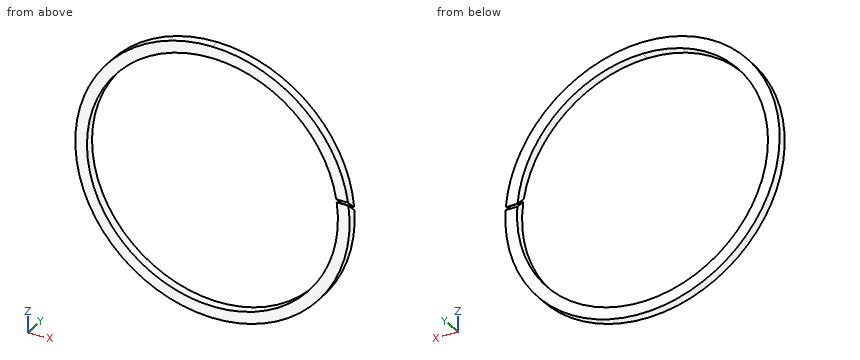
from build123d import *

# Parameters (mm, degrees)
SKETCH1_R           = 47
SKETCH1_R_2         = 43
BOSS_EXTRUDE1_DEPTH = 3
CUT_EXTRUDE1_DEPTH  = 10


with BuildPart() as part:
    # Sketch1 → Boss-Extrude1 (new body)
    with BuildSketch(Plane(origin=(0, 0, 0), x_dir=(1, 0, 0), z_dir=(0, 1, 0))):
        with Locations(Location((0, 0, 0), (0, 0, 270))):
            Circle(SKETCH1_R)
        with Locations(Location((0, 0, 0), (0, 0, 270))):
            Circle(SKETCH1_R_2, mode=Mode.SUBTRACT)
    extrude(amount=BOSS_EXTRUDE1_DEPTH)

    # Sketch3 → Cut-Extrude1 (cut)
    with BuildSketch(Plane(origin=(47, 0, 0), x_dir=(0, 0, -1), z_dir=(1, 0, 0))):
        Polygon((-4, 3), (-7, 0), (-6, 0), (-3, 3), align=None)
    extrude(amount=-CUT_EXTRUDE1_DEPTH, mode=Mode.SUBTRACT)


solid = part.part
Part model, mm, in its own coordinate system. Coordinates: 2 decimals unless noted, no trailing zeros. Order: outer loops, then holes, each group sorted by start corner. A loop starts at its lowest first (then second) coordinate and runs counter-clockwise, first axis right, second up.
(1) Slice it at B-B, the plane x = -37. Write the cut outline in (y, z).
Check sheet entries:
outline: (0, -28.98) - (3, -28.98) - (3, -21.91) - (0, -21.91) - close; (0, 21.91) - (3, 21.91) - (3, 28.98) - (0, 28.98) - close
(2) Slice it at C-C, the plane y = 2.1. Write the cut outline in (x, z), and give its area (3 significant figures).
Check sheet entries:
outline: (42.72, 4.9) - (46.74, 4.9) arc R47 ccw (long way) to (46.84, 3.9) - (42.82, 3.9) arc R43 cw (long way) to start
area: 1,130 mm2
(3) Probe L1, parallel to Z at x = 0, y = 2.4; L2, parallel to Z at x = 7, y = 0.9. List the from-to ranges inside material, lowest first.
Check sheet entries:
L1: z = -47 to -43, 43 to 47
L2: z = -46.48 to -42.43, 42.43 to 46.48
(4) Slice it at A-A, the plane z = 0. Write the cut outline in (x, y).
Check sheet entries:
outline: (-47, 0) - (-43, 0) - (-43, 3) - (-47, 3) - close; (43, 0) - (47, 0) - (47, 3) - (43, 3) - close
